Can you work these out from the model? Positions are in its coordinate system, mm. Face numbers are marked on the shaded views. A direction names the side the tool comes from. Coordinates: 2 decimals unless noted, no trailing zeros. Order: outer loops, then holes, each group sorted by start corner. A loop starts at its lowest first (then second) coordinate and runs counter-clockwise, first axis right, second up. Notation, with made-up numbers: (-16.75, -4.75) -> (38.25, -4.75) arc R15 ccw to (38.25, 11.25) -> close; hole circle Ø1 at (86.5, 74). An arc over 180 degrees is marked (long way). Answer in a Markdown table with one row per item. Add a question column.
1. Will these pins go through, and if not, where does the flat tip stop? pin 1 (12 mm diameter, centred on x = 24.5, y = 11.5, fed in from -Z); pin 2 (1.8 mm diameter, centred on x = 43.04, y = -24.61, fed in from +Z); pin 3 (10 mm diameter, centred on y = 35.5, z = 2, fed in from -X); pin 4 (3.5 mm diameter, centred on y = 26, z = 9.5, fed in from +X).
2. On a 3-axis mill with a long thin cutter (end or side, diameter ignored), from which of +Z, -Z, +X, -X, +Y, -Y can I reach the whole of each face in a straight line? I mean the marked faces 4, 5 and 6. Say none if no direction works.
3. If I drill on line 1 along Y through (x, z) = (65.64, 9.55); line 2 along Z through (x, y) = (9.63, -6.25); line 3 along X through (y, z) = (32.5, -2), over which ranges is the centre line in solid material (lowest first)? Write a range as [from, to].
4. Imagine slicing it at A-A on x = 33.5. State how many separate pieces and enclosed holes the cut face has, plus the area to 3 significant figures.
5. We'd pull the mould along X, two halves only. Please class the marked faces 1, 2 and 3: pulls with the +X half, pulls with the -X half, needs draft (parallel to the pull), parting line crosses it, or undercut.
6. Imagine slicing it at B-B on x = -6. Write out the boundary of the cut face in (y, z).
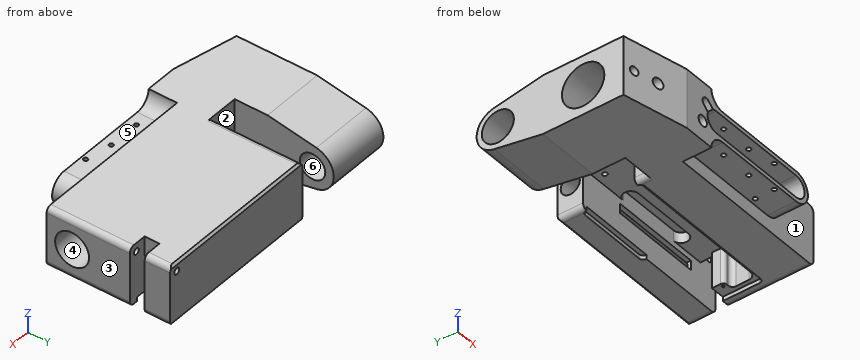
from build123d import *

# Parameters (mm, degrees)
SKETCH1_R                = 1
EXTRUDE1_DEPTH           = 14
CHAMFER1_SIZE            = 1
FILLET1_R                = 2.5
EXTRUDE4_DEPTH           = 30
SKETCH5_R                = 1.5
EXTRUDE5_DEPTH           = 23
SKETCH6_R                = 2.55
SKETCH6_R_2              = 2.05
EXTRUDE6_DEPTH           = 106.731109897
EXTRUDE7_REACH           = 123.359
EXTRUDE8_DEPTH           = 15.49
EXTRUDE21_DEPTH          = 10.11
SKETCH22_R               = 1.2
EXTRUDE22_DEPTH          = 113.348088101
EXTRUDE23_DEPTH          = 113.348088101
EXTRUDE23_DEPTH_BACK     = 8
SKETCH23_R               = 1.2
SKETCH12_R               = 1.5
EXTRUDE12_DEPTH          = 8.5
SKETCH13_R               = 2.5
EXTRUDE13_DEPTH          = 20.48
EXTRUDE14_REACH          = 107.731
EXTRUDE14_END_RADIUS     = 6
SKETCH14_R               = 2.25
SKETCH15_W               = 40.81
SKETCH15_H               = 5
EXTRUDE15_DEPTH          = 20
EXTRUDE24_DEPTH          = 19
EXTRUDE25_DEPTH          = 2
EXTRUDE26_DEPTH          = 5
SKETCH27_R               = 1.25
SKETCH27_R_2             = 1.1
SKETCH27_R_3             = 1
EXTRUDE27_DEPTH          = 6
SKETCH20_R               = 0.6
EXTRUDE20_DEPTH          = 8
CUT_EXTRUDE_1_REACH      = 114.06
CUT_EXTRUDE_1_END_RADIUS = 4.515
SKETCH_1_W               = 42.97
SKETCH_1_H               = 4.52


with BuildPart() as part:
    # Sketch1 → Extrude1 (new, symmetric)
    with BuildSketch(Plane.XY):
        Polygon((0, 0), (0, 46.74), (-30, 46.74), (-30, -22.49), (0, -28.98), (73.21, -28.98), (73.21, -15.51), (93.8, -15.51), (93.8, 23.71), (84.8, 23.71), (84.8, 30.71), (93.8, 30.71), (93.8, 42.75), (13.8, 42.75), (13.8, 0), align=None)
        with Locations((55.55, -17.96)):
            Circle(SKETCH1_R, mode=Mode.SUBTRACT)
        with Locations((55.55, -26.93)):
            Circle(SKETCH1_R, mode=Mode.SUBTRACT)
        with Locations((43.04, -24.61)):
            Circle(SKETCH1_R, mode=Mode.SUBTRACT)
        with Locations((27.87, -24.61)):
            Circle(SKETCH1_R, mode=Mode.SUBTRACT)
    extrude(amount=EXTRUDE1_DEPTH, both=True)

    # Chamfer1
    chamfer1_edges = [part.edges().sort_by_distance(p)[0] for p in [
        (53.8, 42.75, -14),
        (53.8, 42.75, 14),
    ]]
    chamfer(chamfer1_edges, length=CHAMFER1_SIZE)

    # Fillet1
    fillet1_edges = [part.edges().sort_by_distance(p)[0] for p in [
        (13.8, 20.875, -14),
        (93.8, 4.1, -14),
        (93.8, 36.23, -14),
        (93.8, 36.23, 14),
        (93.8, 4.1, 14),
        (13.8, 20.875, 14),
    ]]
    fillet(fillet1_edges, radius=FILLET1_R)

    # Sketch2 → Extrude4 (cut)
    with BuildSketch(Plane.ZY.offset(30)):
        with BuildLine():
            Line((-9.840360705, 38.519691323), (-14, 15.52))
            Line((-14, 15.52), (-14, 50.25246906))
            Line((-14, 50.25246906), (14, 50.25246906))
            Line((14, 50.25246906), (14, 15.52))
            Line((14, 15.52), (9.840360705, 38.519691323))
            ThreePointArc((9.840360705, 38.519691323), (0, 46.74), (-9.840360705, 38.519691323))
        make_face()
    extrude(amount=-EXTRUDE4_DEPTH, mode=Mode.SUBTRACT)

    # Sketch3 → Cut-Revolve1 (revolve, cut)
    with BuildSketch(Plane.XY):
        Polygon((-30, 36.73), (-30, 44.28), (-18.3, 44.28), (-18.3, 42.73), (0, 42.73), (0, 41.245), (13.8, 41.245), (85.68, 41.245), (85.68, 36.73), align=None)
    revolve(axis=Axis((85.68, 36.73, 0), (-1, 0, 0)), mode=Mode.SUBTRACT)

    # Sketch5 → Extrude5 (cut)
    with BuildSketch(Plane(origin=(0, 42.75, 0), x_dir=(1, 0, 0), z_dir=(0, 1, 0))):
        with Locations(Location((89.8, -10, 0), (0, 0, 180))):
            Circle(SKETCH5_R)
    extrude(amount=-EXTRUDE5_DEPTH, mode=Mode.SUBTRACT)

    # Sketch6 → Extrude6 (cut, through all)
    with BuildSketch(Plane(origin=(0, 0, 0), x_dir=(1, 0, 0), z_dir=(0, 1, 0))):
        with Locations(Location((-13.6, 0, 0), (0, 0, 270))):
            Circle(SKETCH6_R)
        with Locations(Location((-24.9, 0, 0), (0, 0, 270))):
            Circle(SKETCH6_R_2)
    extrude(amount=-EXTRUDE6_DEPTH, mode=Mode.SUBTRACT)

    # Extrude7: up to this face of the body (flat: up to its plane)
    extrude7_end = Plane(part.part.faces().sort_by_distance((83.459484326, -15.51, 0))[0])
    # Sketch7 → Extrude7 (cut, up to the picked face)
    with BuildSketch(Plane.XZ.offset(28.98), mode=Mode.PRIVATE) as extrude7_sk1:
        with BuildLine():
            Line((21.69, 7.2), (66.01, 7.2))
            ThreePointArc((66.01, 7.2), (73.21, 0), (66.01, -7.2))
            Line((66.01, -7.2), (21.69, -7.2))
            ThreePointArc((21.69, -7.2), (16.881673888, -9.191673888), (14.89, -14))
            Line((14.89, -14), (80.319549596, -14))
            Line((80.319549596, -14), (80.319549596, 14))
            Line((80.319549596, 14), (14.89, 14))
            ThreePointArc((14.89, 14), (16.881673888, 9.191673888), (21.69, 7.2))
        make_face()
    extrude7_tool1 = split(extrude(extrude7_sk1.sketch, amount=-EXTRUDE7_REACH, mode=Mode.PRIVATE), bisect_by=extrude7_end, keep=Keep.BOTH, mode=Mode.PRIVATE)
    add(extrude7_tool1.solids().sort_by(Axis((47.604775, -28.98, 13.28831), (0, 1, 0)))[0], mode=Mode.SUBTRACT)

    # Sketch8 → Extrude8 (cut)
    with BuildSketch(Plane.XZ.offset(28.98)):
        with BuildLine():
            Line((21.69, 5.2), (66.01, 5.2))
            ThreePointArc((66.01, 5.2), (71.21, 0), (66.01, -5.2))
            Line((66.01, -5.2), (21.69, -5.2))
            Line((21.69, -5.2), (21.69, 5.2))
        make_face()
    extrude(amount=-EXTRUDE8_DEPTH, mode=Mode.SUBTRACT)

    # Sketch9 → Extrude21 (cut)
    with BuildSketch(Plane.XZ.offset(28.98)):
        with BuildLine():
            Line((17.74, 5.2), (21.69, 5.2))
            Line((21.69, 5.2), (21.69, -5.2))
            Line((21.69, -5.2), (17.74, -5.2))
            ThreePointArc((17.74, -5.2), (13.574153864, -3.112189899), (12.753498359, 1.474720781))
            Line((12.753498359, 1.474720781), (10.23607572, 3.741418307))
            ThreePointArc((10.23607572, 3.741418307), (10.070232818, 6.90588939), (13.234703901, 7.071732292))
            Line((13.234703901, 7.071732292), (15.75212654, 4.805034766))
            ThreePointArc((15.75212654, 4.805034766), (16.726634514, 5.100302971), (17.74, 5.2))
        make_face()
    extrude(amount=-EXTRUDE21_DEPTH, mode=Mode.SUBTRACT)

    # Sketch22 → Extrude22 (cut, through all)
    with BuildSketch(Plane.XZ.offset(13.49)):
        with Locations(Location((17.74, 0, 0), (0, 0, 270))):
            Circle(SKETCH22_R)
    extrude(amount=EXTRUDE22_DEPTH, mode=Mode.SUBTRACT)

    # Sketch23 → Extrude23 (cut, two sides: drawn at the far end of the back side and taken through both)
    with BuildSketch(Plane.XZ.offset(13.49).offset(-EXTRUDE23_DEPTH_BACK)):
        with Locations(Location((11.73538981, 5.406575299, 0), (0, 0, 270))):
            Circle(SKETCH23_R)
    extrude(amount=EXTRUDE23_DEPTH + EXTRUDE23_DEPTH_BACK, mode=Mode.SUBTRACT)

    # Sketch12 → Extrude12 (cut)
    with BuildSketch(Plane(origin=(0, 0, 0), x_dir=(1, 0, 0), z_dir=(0, 1, 0))):
        with Locations(Location((9.63, 4.53, 0), (0, 0, 180))):
            Circle(SKETCH12_R)
    extrude(amount=-EXTRUDE12_DEPTH, mode=Mode.SUBTRACT)

    # Sketch13 → Extrude13 (cut)
    with BuildSketch(Plane.XZ.offset(28.98)):
        with Locations(Location((9.63, -4.53, 0), (0, 0, 270))):
            Circle(SKETCH13_R)
    extrude(amount=-EXTRUDE13_DEPTH, mode=Mode.SUBTRACT)

    # Extrude14: up to this cylinder (the profile starts outside it)
    extrude14_end = Plane(origin=(-13.6, 36.73, 0), z_dir=(1, 0, 0)) * Cylinder(EXTRUDE14_END_RADIUS, 228.462, mode=Mode.PRIVATE)
    # Sketch14 → Extrude14 (cut, up to the surface)
    with BuildSketch(Plane(origin=(0, 0, 0), x_dir=(1, 0, 0), z_dir=(0, 1, 0)), mode=Mode.PRIVATE) as extrude14_sk1:
        with Locations(Location((-13.6, 0, 0), (0, 0, 90))):
            Circle(SKETCH14_R)
    extrude14_tool1 = extrude(extrude14_sk1.sketch, amount=EXTRUDE14_REACH, mode=Mode.PRIVATE) - extrude14_end
    add(extrude14_tool1.solids().sort_by_distance((-13.6, 0, 0))[0], mode=Mode.SUBTRACT)

    # Sketch15 → Extrude15 (cut)
    with BuildSketch(Plane.XZ.offset(13.49)):
        with Locations((46.585, 0)):
            Rectangle(SKETCH15_W, SKETCH15_H)
    extrude(amount=-EXTRUDE15_DEPTH, mode=Mode.SUBTRACT)

    # Sketch24 → Extrude24 (cut)
    with BuildSketch(Plane(origin=(0, 0, -14), x_dir=(-1, 0, 0), z_dir=(0, 0, -1))):
        with BuildLine():
            Line((-84.8, 30.71), (-13.8, 30.71))
            Line((-13.8, 30.71), (-13.8, 6.5))
            Line((-13.8, 6.5), (-83.95, 6.5))
            ThreePointArc((-83.95, 6.5), (-86.332949853, 7.487050147), (-87.32, 9.87))
            Line((-87.32, 9.87), (-87.32, 15.96))
            ThreePointArc((-87.32, 15.96), (-86.716639969, 17.416639969), (-85.26, 18.02))
            Line((-85.26, 18.02), (-84.47, 18.02))
            ThreePointArc((-84.47, 18.02), (-83.27498954, 18.51498954), (-82.78, 19.71))
            Line((-82.78, 19.71), (-82.78, 23.71))
            Line((-82.78, 23.71), (-84.8, 23.71))
            Line((-84.8, 23.71), (-84.8, 30.71))
        make_face()
    extrude(amount=-EXTRUDE24_DEPTH, mode=Mode.SUBTRACT)

    # Sketch25 → Extrude25 (cut)
    with BuildSketch(Plane(origin=(0, 0, -14), x_dir=(-1, 0, 0), z_dir=(0, 0, -1))):
        with BuildLine():
            Line((-15.8, 6.5), (-15.8, 23.71))
            Line((-15.8, 23.71), (-89.32, 23.71))
            Line((-89.32, 23.71), (-89.32, 6.5))
            ThreePointArc((-89.32, 6.5), (-88.734213562, 5.085786438), (-87.32, 4.5))
            Line((-87.32, 4.5), (-17.8, 4.5))
            ThreePointArc((-17.8, 4.5), (-16.385786438, 5.085786438), (-15.8, 6.5))
        make_face()
        with BuildLine():
            Line((-17.8, 32.71), (-50.14, 32.71))
            ThreePointArc((-50.14, 32.71), (-51.554213562, 32.124213562), (-52.14, 30.71))
            Line((-52.14, 30.71), (-52.14, 28.71))
            Line((-52.14, 28.71), (-15.8, 28.71))
            Line((-15.8, 28.71), (-15.8, 30.71))
            ThreePointArc((-15.8, 30.71), (-16.385786438, 32.124213562), (-17.8, 32.71))
        make_face()
    extrude(amount=-EXTRUDE25_DEPTH, mode=Mode.SUBTRACT)

    # Sketch26 → Extrude26 (cut)
    with BuildSketch(Plane(origin=(0, 0, 5), x_dir=(-1, 0, 0), z_dir=(0, 0, -1))):
        with BuildLine():
            Line((-38.25, 30.71), (-68.47, 30.71))
            ThreePointArc((-68.47, 30.71), (-71.97, 27.21), (-68.47, 23.71))
            Line((-68.47, 23.71), (-38.25, 23.71))
            ThreePointArc((-38.25, 23.71), (-34.75, 27.21), (-38.25, 30.71))
        make_face()
    extrude(amount=-EXTRUDE26_DEPTH, mode=Mode.SUBTRACT)

    # Sketch4 → Cut-Revolve2 (revolve, cut)
    with BuildSketch(Plane.XY, mode=Mode.PRIVATE) as cut_revolve2_sk:
        Polygon((-32.954746832, 6.51), (-32.954746832, -3.49), (100.534470899, -3.49), (100.534470899, 4.51), (21.600016289, 4.51), (21.600016289, -0.99), (-1.117704794, -0.99), (-1.117704794, 6.51), align=None)
    revolve(cut_revolve2_sk.sketch.rotate(Axis((-36.156901719, -3.49, 0), (1, 0, 0)), 90), axis=Axis((-36.156901719, -3.49, 0), (1, 0, 0)), mode=Mode.SUBTRACT)

    # Sketch27 → Extrude27 (cut)
    with BuildSketch(Plane(origin=(0, 0, 5), x_dir=(-1, 0, 0), z_dir=(0, 0, -1))):
        with Locations((-65.64, 11.33)):
            Circle(SKETCH27_R)
        with Locations((-21.56, 26.46)):
            Circle(SKETCH27_R_2)
        with Locations((-85.26, 15.96)):
            Circle(SKETCH27_R_3)
        with Locations((-42.01, 11.33)):
            Circle(SKETCH27_R)
    extrude(amount=-EXTRUDE27_DEPTH, mode=Mode.SUBTRACT)

    # Sketch20 → Extrude20 (cut)
    with BuildSketch(Plane.XY.offset(-12)):
        with Locations((84.47, 19.71)):
            Circle(SKETCH20_R)
    extrude(amount=EXTRUDE20_DEPTH, mode=Mode.SUBTRACT)

    # 切除-拉伸1: up to this cylinder (the profile starts outside it)
    cut_extrude_1_end = Plane(origin=(57.535, 36.73, 0), z_dir=(1, 0, 0)) * Cylinder(CUT_EXTRUDE_1_END_RADIUS, 238.15, mode=Mode.PRIVATE)
    # 草图1 → 切除-拉伸1 (cut, up to the surface)
    with BuildSketch(Plane.XZ.offset(-30.71), mode=Mode.PRIVATE) as cut_extrude_1_sk1:
        with Locations((57.535, 0)):
            Rectangle(SKETCH_1_W, SKETCH_1_H)
    cut_extrude_1_tool1 = extrude(cut_extrude_1_sk1.sketch, amount=-CUT_EXTRUDE_1_REACH, mode=Mode.PRIVATE) - cut_extrude_1_end
    add(cut_extrude_1_tool1.solids().sort_by_distance((57.535, 30.71, 0))[0], mode=Mode.SUBTRACT)


solid = part.part
Answers follow:
| question | item | result |
|---|---|---|
| 1 | pin 1 | stops at z = -12 |
| 1 | pin 2 | passes through |
| 1 | pin 3 | stops at x = -18.3 |
| 1 | pin 4 | stops at x = 84.8 |
| 2 | face 4 | +X |
| 2 | face 5 | +Z, +X, -Y |
| 2 | face 6 | -X |
| 3 | line 1 | y = [-15.51, 10.08], [12.58, 23.71], [30.71, 42.75] |
| 3 | line 2 | z = [-14, -6.03], [-3.03, 14] |
| 3 | line 3 | x = [13.8, 36.05], [79.02, 93.8] |
| 4 | separate pieces | 2 |
| 4 | enclosed holes | 1 |
| 4 | area | 909 mm² |
| 5 | face 1 | needs draft |
| 5 | face 2 | undercut |
| 5 | face 3 | pulls with the +X half |
| 6 | outline | (-27.68, -14) -> (15.52, -14) -> (38.52, -9.84) arc R10 ccw to (38.52, 9.84) -> (15.52, 14) -> (-27.68, 14) -> close; hole circle Ø20 at (-3.49, 0); hole circle Ø12 at (36.73, 0) |
